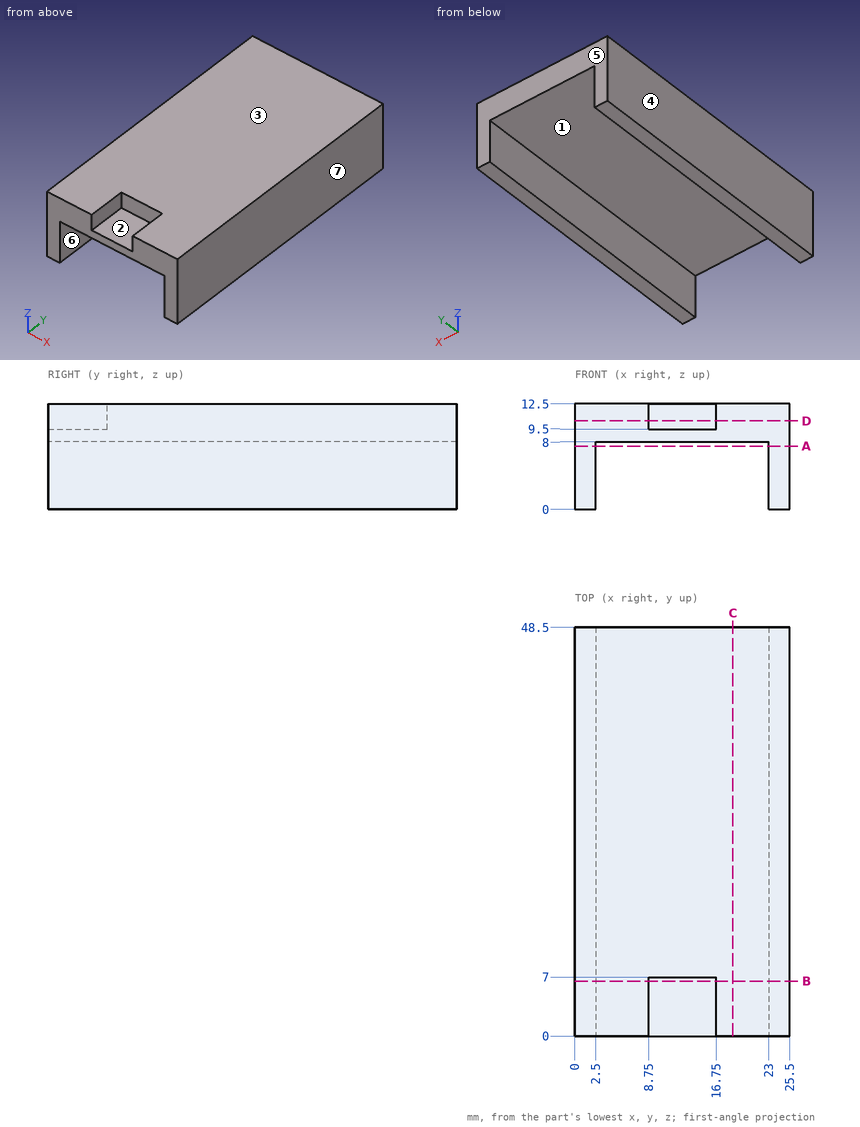
Geometry check sheet. Reference: drawing and pictorial views, mm from the part's lowest x, y, z. A direction names the side the tool comes from. Round coordinates to 2 decimals unless told otherwise and drop trailing zeros. Order: outer loops, then holes, each group sorted by start corner. A loop starts at its lowest first (then second) coordinate and runs counter-clockwise, first axis right, second up. Notation, with made-up numbers: (-5.75, -33.75) - (1.25, -33.75) arc R11 ccw to (1.25, -21.75) - close; hole circle Ø4 at (30.25, -29). An arc over 180 degrees is marked (long way). Use a Markdown table: item, result. Add a question column.
1) Thickness scan on line 1 along X through (y, z) = (25, 4); line 2 along Z through (x, y) = (16, 20); line 3 along X through (y, z) = (5.5, 12). Record the ranges inside material, lowest first.
2) Section check A-A (z = 7.5). Record the cut outline in (x, y).
3) Section check C-C (x = 18.75). Record the cut outline in (y, z), then the cut area to 3 significant figures.
4) Section check D-D (z = 10.5). Record the cut outline in (x, y).
5) Mould release check, pull along X, two halves, no side actions. Record for the marked faces 4, 5, 6 and 7: released by +X, released by -X, zero draft, split by the parting line, or undercut.
6) Section check B-B (y = 6.5). Record the cut outline in (x, z).
7) Set-up check for the marked faces 1, 2 and 3: record each of +Z, -Z, +X, -X, +Y, -Y from which the full face is reachable in a straight line by a thin tool's end or side.
8) Gauge pin test, flat ends, axial feed: P1, Ø1.5, axis at x = 5, z = 2, coming from the +Y side (3 decimals); P2, Ø0.9, axis at x = 12.5, z = 10.5, coming from the -Y side. Record the tip position at first contact, or that the pin passes through.
Established:
| question | item | result |
|---|---|---|
| 1 | line 1 | 0 to 2.5, 23 to 25.5 |
| 1 | line 2 | 8 to 12.5 |
| 1 | line 3 | 0 to 8.75, 16.75 to 25.5 |
| 2 | outline | (0, 0) - (2.5, 0) - (2.5, 48.5) - (0, 48.5) - close; (23, 0) - (25.5, 0) - (25.5, 48.5) - (23, 48.5) - close |
| 3 | outline | (0, 8) - (48.5, 8) - (48.5, 12.5) - (0, 12.5) - close |
| 3 | area | 218 mm2 |
| 4 | outline | (0, 0) - (8.75, 0) - (8.75, 7) - (16.75, 7) - (16.75, 0) - (25.5, 0) - (25.5, 48.5) - (0, 48.5) - close |
| 5 | face 4 | released by -X |
| 5 | face 5 | zero draft |
| 5 | face 6 | undercut |
| 5 | face 7 | released by +X |
| 6 | outline | (0, 0) - (2.5, 0) - (2.5, 8) - (23, 8) - (23, 0) - (25.5, 0) - (25.5, 12.5) - (16.75, 12.5) - (16.75, 9.5) - (8.75, 9.5) - (8.75, 12.5) - (0, 12.5) - close |
| 7 | face 1 | -Z, +Y, -Y |
| 7 | face 2 | +Z, -Y |
| 7 | face 3 | +Z, +X, -X, +Y, -Y |
| 8 | P1 | through |
| 8 | P2 | y = 7 |
